```python
from build123d import *

# Parameters (mm, degrees)
SKETCH1_W                      = 20
SKETCH1_H                      = 20
BOSS_EXTRUDE1_DEPTH            = 2
BOSS_EXTRUDE3_DEPTH            = 1.5
BOSS_EXTRUDE3_DEPTH_BACK       = 3.5
TAP_DRILL_FOR_M2_2_HELICOIL1_D = 6.5


with BuildPart() as part:
    # Sketch1 → Boss-Extrude1 (new body)
    with BuildSketch(Plane(origin=(0, 0, 0), x_dir=(1, 0, 0), z_dir=(0, 1, 0))):
        Rectangle(SKETCH1_W, SKETCH1_H)
    extrude(amount=BOSS_EXTRUDE1_DEPTH)

    # Sketch3 → Boss-Extrude3 (add, two sides: drawn at the far end of the back side and taken through both)
    with BuildSketch(Plane(origin=(0, 2, 0), x_dir=(1, 0, 0), z_dir=(0, 1, 0)).offset(-BOSS_EXTRUDE3_DEPTH_BACK)):
        Polygon((-2.875, 8.25), (2.875, 8.25), (2.875, 2.867474963), (8.25, 2.867474963), (8.25, -2.882525037), (2.875, -2.875), (2.875, -8.25), (-2.875, -8.25), (-2.875, -2.875), (-8.25, -2.875), (-8.25, 2.875), (-2.875, 2.875), align=None)
    extrude(amount=BOSS_EXTRUDE3_DEPTH + BOSS_EXTRUDE3_DEPTH_BACK)

    # Tap Drill for M2.2 Helicoil1 (through all)
    with Locations(Plane.ZX.offset(3.5)):
        with Locations((0, 0)):
            Hole(TAP_DRILL_FOR_M2_2_HELICOIL1_D / 2)


solid = part.part
```
Design review of the part built by this model. Coordinates are the model's own, in mm. A direction names the side the tool comes from. Round coordinates to 2 decimals unless told otherwise and drop trailing zeros. Write each loop counter-clockwise with the first axis right and the second up, starting at its lowest first coordinate (ties: lowest second). Pieces come first, ordered by that corner, then holes.
Item 1: For faces 1 (the flat face through (0, -1, 8.25)), 2 (the flat face through (-6, -1, -2.875)), 3 (the flat face through (6, -1, -2.867)), 4 (the flat face through (0, 3, -8.25)), list the 3-axis set-ups (+Z, -Z, +X, -X, +Y, -Y) from which the entire face can be reached by the end or side of a thin tool; tool diameter is ignored.
Item 2: We need section D-D on z = -5. Write out the cut boundary in (x, y) (3 decimals), and give its area (4 significant figures).
Item 3: For probe 1 along X at (y, z) = (-0.2, 0); probe 2 along X at (y, z) = (1.5, 0); probe 3 along Y at (x, z) = (-8.75, 4.5), list the stretches that pass through material, from the lowest coordinate up.
Item 4: Clearance check with flat-ended pins moving along their axes: pin 1 Ø3 at (y, z) = (2.5, 5) entering from -X; pin 2 Ø1.2 at (y, z) = (-1, 5.5) entering from -X (3 decimals); pin 3 Ø0.8 at (x, y) = (1, 3) entering from -Z; pin 4 Ø1.2 at (y, z) = (-1, -0.5) entering from -X. State where each tip first meets the part, or that it passes through.
Item 5: We need section C-C on y = 1.5. Write out the cut boundary in (x, z), and give its area (3 significant figures).
Item 6: We need section A-A on x = 0. Write out the cut boundary in (y, z).
Item 7: We need section B-B on z = 0. Write out the cut boundary in (x, y).
Returned:
1. face 1: +Z, +X, -X, -Y
1. face 2: -Z, -X, -Y
1. face 3: -Z, +X, -Y
1. face 4: -Z, +X, -X, +Y
2. outline: (-10, 0) - (-2.875, 0) - (-2.875, -1.5) - (2.875, -1.5) - (2.875, 0) - (10, 0) - (10, 2) - (2.875, 2) - (2.875, 3.5) - (-2.875, 3.5) - (-2.875, 2) - (-10, 2) - close
2. area: 57.25 mm2
3. probe 1: x = -8.25 to -3.25, 3.25 to 8.25
3. probe 2: x = -10 to -3.25, 3.25 to 10
3. probe 3: y = 0 to 2
4. pin 1: stops at x = -10
4. pin 2: stops at x = -2.875
4. pin 3: stops at z = -8.25
4. pin 4: stops at x = -8.25
5. outline: (-10, -10) - (10, -10) - (10, 10) - (-10, 10) - close; hole circle Ø6.5 at (0, 0)
5. area: 367 mm2
6. outline: (-1.5, -8.25) - (0, -8.25) - (0, -10) - (2, -10) - (2, -8.25) - (3.5, -8.25) - (3.5, -3.25) - (-1.5, -3.25) - close; (-1.5, 3.25) - (3.5, 3.25) - (3.5, 8.25) - (2, 8.25) - (2, 10) - (0, 10) - (0, 8.25) - (-1.5, 8.25) - close
7. outline: (-10, 0) - (-8.25, 0) - (-8.25, -1.5) - (-3.25, -1.5) - (-3.25, 3.5) - (-8.25, 3.5) - (-8.25, 2) - (-10, 2) - close; (3.25, -1.5) - (8.25, -1.5) - (8.25, 0) - (10, 0) - (10, 2) - (8.25, 2) - (8.25, 3.5) - (3.25, 3.5) - close
